```python
from build123d import *

# Parameters (mm, degrees)
SKETCH1_W           = 165
SKETCH1_H           = 30
BOSS_EXTRUDE1_DEPTH = 40
FILLET1_R           = 15
SKETCH2_W           = 26
SKETCH2_H           = 7
BOSS_EXTRUDE2_DEPTH = 6
SKETCH3_R           = 4
BOSS_EXTRUDE3_DEPTH = 10


with BuildPart() as part:
    # Sketch1 → Boss-Extrude1 (new body)
    with BuildSketch(Plane.XY):
        Rectangle(SKETCH1_W, SKETCH1_H)
    extrude(amount=BOSS_EXTRUDE1_DEPTH)

    # Fillet1
    fillet1_edges = [part.edges().sort_by_distance(p)[0] for p in [
        (-82.5, 15, 20),
        (82.5, -15, 20),
        (-82.5, -15, 20),
        (82.5, 15, 20),
    ]]
    fillet(fillet1_edges, radius=FILLET1_R - 0.0001)  # a hair under: the kernel refuses the full size

    # Sketch2 → Boss-Extrude2 (add)
    with BuildSketch(Plane.XZ.offset(15)):
        with Locations((0, 10.5)):
            Rectangle(SKETCH2_W, SKETCH2_H)
    extrude(amount=BOSS_EXTRUDE2_DEPTH)

    # Sketch3 → Boss-Extrude3 (add)
    with BuildSketch(Plane.XY.offset(40)):
        with Locations((0, -4)):
            Circle(SKETCH3_R)
    extrude(amount=BOSS_EXTRUDE3_DEPTH)


solid = part.part
```
Check sheet for the modelled part. Datum: model origin and axes. Units: mm. A direction names the side the tool comes from. Coordinates: 2 decimals unless noted, no trailing zeros. Order: outer loops, then holes, each group sorted by start corner. A loop starts at its lowest first (then second) coordinate and runs counter-clockwise, first axis right, second up. Notation, with made-up numbers: M 26.25,86 L 79.25,86 A11 ccw 79.25,93 Z; hole C -21,-37.75 d10. An arc over 180 degrees is marked long. One line per question, with ' | ' between items. Start each with the question number.
Item 1: Material ranges on line 1 (Z direction, x = 50, y = -4); line 2 (Y direction, x = -7, z = 27); line 3 (X direction, y = 8.5, z = 15), recorded low to high.
Item 2: Sectioned sample at B-B on x = -6.5. Record the cut outline in (y, z).
Item 3: Gauge pin test, flat ends, axial feed: P1, Ø4, axis at y = -2, z = 29.5, coming from the -X side; P2, Ø1, axis at x = 29, y = -8.5, coming from the +Z side; P3, Ø1, axis at x = -24, z = 10, coming from the -Y side; P4, Ø1.8, axis at y = -19, z = 11.5, coming from the -X side. Record the tip position at first contact, or that the pin passes through.
Item 4: Sectioned sample at D-D on y = 5.5. Record the cut outline in (x, z), and give its area (3 significant figures).
Item 5: Access from +Z, -Z, +X, -X, +Y, -Y to the whole of each face (thin tool, end or side, straight path). Record for faces 1 (the flat face through (0, -18, 7)), 2 (the flat face through (13, -18, 10)), 3 (the flat face through (0, -18, 14)), 4 (the cylindrical face through (-0.867, -7.905, 44.93)).
Answer below:
1) line 1: z = 0 to 40 | line 2: y = -15 to 15 | line 3: x = -79.86 to 79.86
2) outline: M -21,7 L -15,7 L -15,0 L 15,0 L 15,40 L -15,40 L -15,14 L -21,14 Z
3) P1: stops at x = -82.5 | P2: stops at z = 40 | P3: stops at y = -15 | P4: stops at x = -13
4) outline: M -81.46,0 L 81.46,0 L 81.46,40 L -81.46,40 Z | area: 6,520 mm^2
5) face 1: -Z, +X, -X, -Y | face 2: +Z, -Z, +X, -Y | face 3: +Z, +X, -X, -Y | face 4: +Z
